Verification items for the finished model (mm, model axes). Face numbers are marked on the shaded views. A direction names the side the tool comes from. Give positions to 0.01 mm unless a question says otherwise; leave off trailing zeros. Order: outer loops, then holes, each group sorted by start corner. A loop starts at its lowest first (then second) coordinate and runs counter-clockwise, first axis right, second up. Notation, with made-up numbers: (-11.75, -9.75) -> (-7.75, -9.75) arc R23 ccw to (-7.75, 12.25) -> close; hole circle Ø1 at (37, -14.5). An arc over 180 degrees is marked (long way). Return JSON: item names as keys, results as strings. Group by question number.
(1) Depth check by flat-ended pin: pin 1 Ø10 at (x, z) = (134.5, -7) entering from +Y; pin 2 Ø8 at (x, y) = (-68.5, 149) entering from -Z; pin 3 Ø4 at (x, y) = (107, 482.5) entering from +Z. Enter the tip coordinate at first touch or a pass-through.
(2) Thickness scan on line 1 along X through (y, z) = (256, 1); line 2 along Z through (x, y) = (130, 218); line 3 along Z through (x, y) = (134, 167). Record the ranges inside material, lowest first.
(3) Cross-section at D-D on z = -40. State how many separate pieces and enclosed holes the cut face has, then the cut area to 3 significant figures.
(4) Tool access check on the marked faces 1, 2 and 3. Record the directions out of +Z, -Z, +X, -X, +Y, -Y that give a thin tool (end or side, any length) a straight path to the whole face; none if there is none.
(5) Cross-section at A-A on y = 66.04. Enter the section's corners in (x, z).
(6) Cross-section at C-C on y = -33.5. Enter the section's corners in (x, z), then the cut area to 3 significant figures.
(7) Cross-section at B-B on x = 0. Enter the section's corners in (y, z).
from build123d import *

# Parameters (mm, degrees)
SIDE_PROFILE_EXTRUDE_DEPTH             = 6.35
MOUNTING_BRACKET_PROFILE_SKETCH_W      = 152.4
MOUNTING_BRACKET_PROFILE_SKETCH_H      = 508
MOUNTING_BRACKET_PROFILE_EXTRUDE_DEPTH = 12.7
MOUNTING_BRACKET_HOLES_SKETCH_R        = 12.7
MOUNTING_BRACKET_HOLES_CUT_DEPTH       = 12.7
OUTER_TRACK_CUT_DEPTH                  = 12.7
INNER_TRACK_CUT_DEPTH                  = 12.7


with BuildPart() as part:
    # Side Profile Sketch → Side Profile Extrude (new, symmetric)
    with BuildSketch(Plane.XY):
        with BuildLine():
            Line((-127, 0), (-127, 508))
            ThreePointArc((-127, 508), (0, 635), (127, 508))
            Line((127, 508), (127, 0))
            ThreePointArc((127, 0), (0, -127), (-127, 0))
        make_face()
    extrude(amount=SIDE_PROFILE_EXTRUDE_DEPTH, both=True)

    # Mounting Bracket Profile Sketch → Mounting Bracket Profile Extrude (add)
    with BuildSketch(Plane(origin=(127, 0, 0), x_dir=(0, 0, -1), z_dir=(1, 0, 0))):
        with Locations((0, 254)):
            Rectangle(MOUNTING_BRACKET_PROFILE_SKETCH_W, MOUNTING_BRACKET_PROFILE_SKETCH_H)
    extrude(amount=MOUNTING_BRACKET_PROFILE_EXTRUDE_DEPTH)

    # Mounting Bracket Holes Sketch → Mounting Bracket Holes Cut (cut)
    with BuildSketch(Plane(origin=(139.7, 0, 0), x_dir=(0, 0, -1), z_dir=(1, 0, 0))):
        with Locations((-40.64, 472.44)):
            Circle(MOUNTING_BRACKET_HOLES_SKETCH_R)
        with Locations((-40.64, 421.64)):
            Circle(MOUNTING_BRACKET_HOLES_SKETCH_R)
        with Locations((-40.64, 370.84)):
            Circle(MOUNTING_BRACKET_HOLES_SKETCH_R)
        with Locations((-40.64, 320.04)):
            Circle(MOUNTING_BRACKET_HOLES_SKETCH_R)
        with Locations((-40.64, 269.24)):
            Circle(MOUNTING_BRACKET_HOLES_SKETCH_R)
        with Locations((-40.64, 218.44)):
            Circle(MOUNTING_BRACKET_HOLES_SKETCH_R)
        with Locations((-40.64, 167.64)):
            Circle(MOUNTING_BRACKET_HOLES_SKETCH_R)
        with Locations((-40.64, 116.84)):
            Circle(MOUNTING_BRACKET_HOLES_SKETCH_R)
        with Locations((-40.64, 66.04)):
            Circle(MOUNTING_BRACKET_HOLES_SKETCH_R)
        with Locations((40.64, 66.04)):
            Circle(MOUNTING_BRACKET_HOLES_SKETCH_R)
        with Locations((40.64, 116.84)):
            Circle(MOUNTING_BRACKET_HOLES_SKETCH_R)
        with Locations((40.64, 167.64)):
            Circle(MOUNTING_BRACKET_HOLES_SKETCH_R)
        with Locations((40.64, 218.44)):
            Circle(MOUNTING_BRACKET_HOLES_SKETCH_R)
        with Locations((40.64, 269.24)):
            Circle(MOUNTING_BRACKET_HOLES_SKETCH_R)
        with Locations((40.64, 320.04)):
            Circle(MOUNTING_BRACKET_HOLES_SKETCH_R)
        with Locations((40.64, 370.84)):
            Circle(MOUNTING_BRACKET_HOLES_SKETCH_R)
        with Locations((40.64, 421.64)):
            Circle(MOUNTING_BRACKET_HOLES_SKETCH_R)
        with Locations((40.64, 472.44)):
            Circle(MOUNTING_BRACKET_HOLES_SKETCH_R)
    extrude(amount=-MOUNTING_BRACKET_HOLES_CUT_DEPTH, mode=Mode.SUBTRACT)

    # Outer Track Sketch → Outer Track Cut (cut)
    with BuildSketch(Plane.XY.offset(6.35)):
        with BuildLine():
            Line((-107.95, 0), (-107.95, 508))
            ThreePointArc((-107.95, 508), (0, 615.95), (107.95, 508))
            Line((107.95, 508), (95.25, 508))
            ThreePointArc((95.25, 508), (0, 603.25), (-95.25, 508))
            Line((-95.25, 508), (-95.25, 0))
            ThreePointArc((-95.25, 0), (0, -95.25), (95.25, 0))
            Line((95.25, 0), (107.95, 0))
            ThreePointArc((107.95, 0), (0, -107.95), (-107.95, 0))
        make_face()
    extrude(amount=-OUTER_TRACK_CUT_DEPTH, mode=Mode.SUBTRACT)

    # Inner Track Sketch → Inner Track Cut (cut)
    with BuildSketch(Plane.XY.offset(6.35)):
        with BuildLine():
            Line((-57.15, 0), (-57.15, 508))
            ThreePointArc((-57.15, 508), (0, 565.15), (57.15, 508))
            Line((57.15, 508), (44.45, 508))
            ThreePointArc((44.45, 508), (0, 552.45), (-44.45, 508))
            Line((-44.45, 508), (-44.45, 0))
            ThreePointArc((-44.45, 0), (0, -44.45), (44.45, 0))
            Line((44.45, 0), (57.15, 0))
            ThreePointArc((57.15, 0), (0, -57.15), (-57.15, 0))
        make_face()
    extrude(amount=-INNER_TRACK_CUT_DEPTH, mode=Mode.SUBTRACT)


solid = part.part
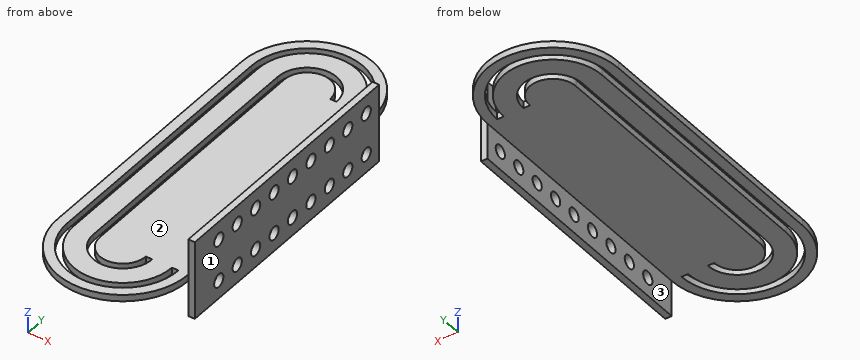
Verdict:
{
 "1": {"pin 1": "y = 508", "pin 2": "z = -6.35", "pin 3": "z = 6.35"},
 "2": {"line 1": "-127 to -107.95, -95.25 to -57.15, -44.45 to 139.7", "line 2": "-76.2 to -53.33, -27.95 to 27.95, 53.33 to 76.2", "line 3": "-76.2 to -53.32, -27.96 to 27.96, 53.32 to 76.2"},
 "3": {"separate pieces": "10", "enclosed holes": "0", "area": "3,550 mm²"},
 "4": {"face 1": "+Z, -Z, +X, +Y, -Y", "face 2": "+Z, -X, +Y, -Y", "face 3": "-Z, -X, +Y, -Y"},
 "5": {"outline": "(-127, -6.35) -> (-107.95, -6.35) -> (-107.95, 6.35) -> (-127, 6.35) -> close; (-95.25, -6.35) -> (-57.15, -6.35) -> (-57.15, 6.35) -> (-95.25, 6.35) -> close; (-44.45, -6.35) -> (127, -6.35) -> (127, -27.94) -> (139.7, -27.94) -> (139.7, 27.94) -> (127, 27.94) -> (127, 6.35) -> (-44.45, 6.35) -> close; (127, -76.2) -> (139.7, -76.2) -> (139.7, -53.34) -> (127, -53.34) -> close; (127, 53.34) -> (139.7, 53.34) -> (139.7, 76.2) -> (127, 76.2) -> close"},
 "6": {"outline": "(-122.5, -6.35) -> (-102.62, -6.35) -> (-102.62, 6.35) -> (-122.5, 6.35) -> close; (-89.16, -6.35) -> (-46.3, -6.35) -> (-46.3, 6.35) -> (-89.16, 6.35) -> close; (-29.22, -6.35) -> (29.22, -6.35) -> (29.22, 6.35) -> (-29.22, 6.35) -> close; (46.3, -6.35) -> (89.16, -6.35) -> (89.16, 6.35) -> (46.3, 6.35) -> close; (102.62, -6.35) -> (122.5, -6.35) -> (122.5, 6.35) -> (102.62, 6.35) -> close", "area": "2,340 mm²"},
 "7": {"outline": "(-127, -6.35) -> (-107.95, -6.35) -> (-107.95, 6.35) -> (-127, 6.35) -> close; (-95.25, -6.35) -> (-57.15, -6.35) -> (-57.15, 6.35) -> (-95.25, 6.35) -> close; (-44.45, -6.35) -> (552.45, -6.35) -> (552.45, 6.35) -> (-44.45, 6.35) -> close; (565.15, -6.35) -> (603.25, -6.35) -> (603.25, 6.35) -> (565.15, 6.35) -> close; (615.95, -6.35) -> (635, -6.35) -> (635, 6.35) -> (615.95, 6.35) -> close"}
}
